Part print with two shaded views. Sizes in mm from the minimum x, y, z corner. A direction names the side the tool comes from. Give positions to 0.01 mm unless a question says otherwise; leave off trailing zeros. Loops run counter-clockwise (first coordinate to the right, second up) from the corner with the lowest first, then second, coordinate; pieces in that order, holes last. Notation, with made-up numbers: (-7.5, 5) -> (39.5, 5) arc R10 cw to (39.5, 19) -> close; hole circle Ø8 at (-18, -33). An arc over 180 degrees is marked (long way). One line per question, with ' | ' between items. Start each with the question number.
(1) Slice it at B-B, the plane y = 48.5. Write the cut outline in (x, z).
(2) 3-axis set-ups, long thin cutter, end or side, ignore diameter. For the marked faces 1, 2 and 3: which of +Z, -Z, +X, -X, +Y, -Y reach the whole face in a straight line?
(3) Slice it at D-D, the plane y = 38.5. Write the cut outline in (x, z).
(4) Slice it at A-A, the plane x = 15.5. Write the cut outline in (y, z), then the cut area to 3 significant figures.
(5) Drill centre lines: L1, parallel to Z at x = 9.75, y = 33; L2, parallel to Y at x = 7.5, z = 10.25; L3, parallel to Y at x = 15.5, z = 0.6. Where is each one in solid material? Low to high. Write a range as from..to.
(6) Slice it at C-C, the plane x = 13. Write the cut outline in (y, z).
(7) Flat gauge pins, fed straight in: pin 1 Ø1 at (x, z) = (13.5, 9.5) entering from -Y; pin 2 Ø2 at (x, y) = (8.5, 49.5) entering from +Z; pin 3 Ø12 at (x, y) = (3, 11) entering from -Z; pin 4 Ø5 at (y, z) = (37.5, 15) entering from +X. Where does each tip first touch, or does it go through?
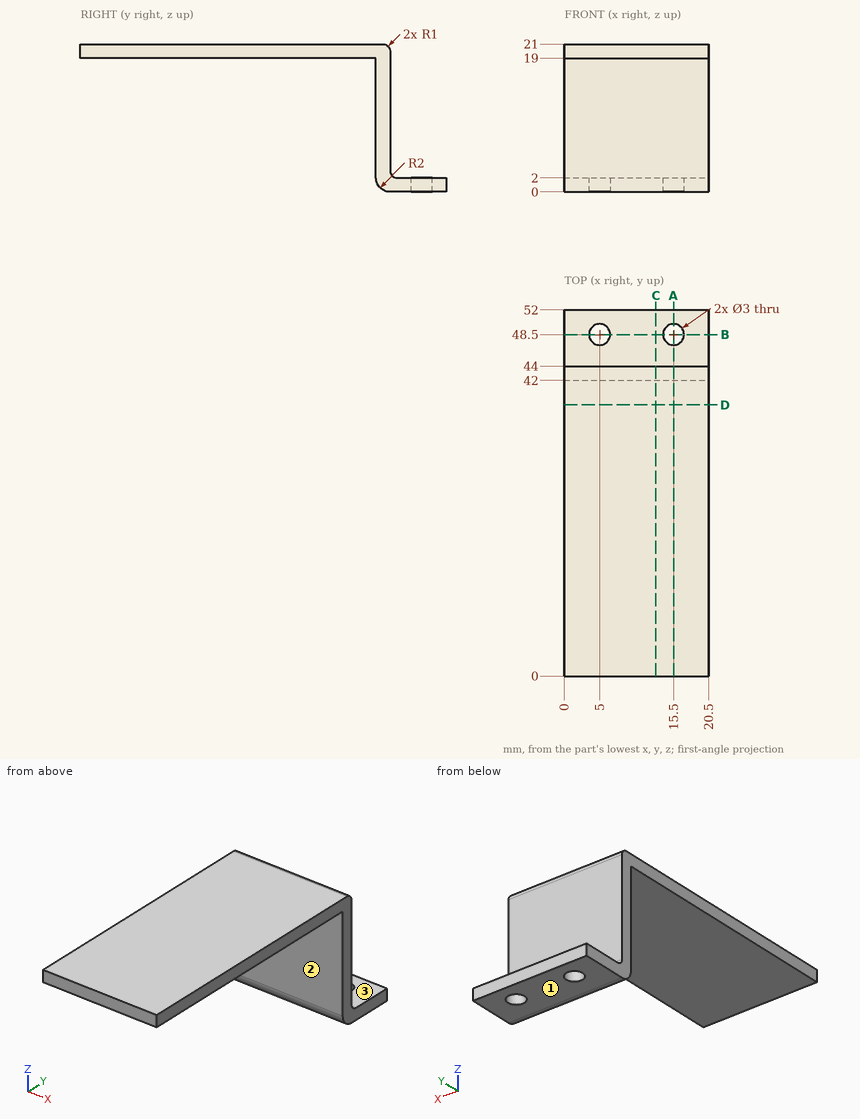
Final values:
1) outline: (0, 0) -> (3.5, 0) -> (3.5, 2) -> (0, 2) -> close; (6.5, 0) -> (14, 0) -> (14, 2) -> (6.5, 2) -> close; (17, 0) -> (20.5, 0) -> (20.5, 2) -> (17, 2) -> close
2) face 1: -Z, +X, -X, +Y, -Y | face 2: -Z, +X, -X, -Y | face 3: +Z, +X, -X, +Y
3) outline: (0, 19) -> (20.5, 19) -> (20.5, 21) -> (0, 21) -> close
4) outline: (0, 19) -> (42, 19) -> (42, 2) arc R2 ccw to (44, 0) -> (47, 0) -> (47, 2) -> (45, 2) arc R1 cw to (44, 3) -> (44, 20) arc R1 ccw to (43, 21) -> (0, 21) -> close; (50, 0) -> (52, 0) -> (52, 2) -> (50, 2) -> close | area: 135 mm2
5) L1: 19..21 | L2: 42..44 | L3: 42.57..47, 50..52
6) outline: (0, 19) -> (42, 19) -> (42, 2) arc R2 ccw to (44, 0) -> (52, 0) -> (52, 2) -> (45, 2) arc R1 cw to (44, 3) -> (44, 20) arc R1 ccw to (43, 21) -> (0, 21) -> close
7) pin 1: y = 42 | pin 2: z = 2 | pin 3: z = 19 | pin 4: through
